from build123d import *

# Parameters (mm, degrees)
ESQUISSE2_W             = 5
ESQUISSE2_H             = 12.5
ESQUISSE3_R             = 2
ENL_V_MAT_EXTRU_1_DEPTH = 36
ESQUISSE4_R             = 3
ENL_V_MAT_EXTRU_2_DEPTH = 36
ESQUISSE5_W             = 30
ESQUISSE5_H             = 3.421913798


with BuildPart() as part:
    # Esquisse1 → Révolution1 (revolve)
    with BuildSketch(Plane.XY):
        Polygon((0, 34), (0, 0), (8, 0), (8, 40), (3, 40), (3, 39), (-27, 39), (-27, 40), (-32, 40), (-32, 34), align=None)
    revolve(axis=Axis((-49.644499027, 0, 0), (1, 0, 0)))

    # Esquisse2 → Enlèvement de matière-Révolution1 (revolve, cut)
    with BuildSketch(Plane.XY):
        with Locations((5.5, 6.25)):
            Rectangle(ESQUISSE2_W, ESQUISSE2_H)
    revolve(axis=Axis((0, 0, 0), (1, 0, 0)), mode=Mode.SUBTRACT)

    # Esquisse3 → Enlèv. mat.-Extru.1 (cut, through all)
    with BuildSketch(Plane(origin=(3, 0, 0), x_dir=(0, 0, -1), z_dir=(1, 0, 0))):
        with Locations((4.75, 8.227241336)):
            Circle(ESQUISSE3_R)
        with Locations((-4.75, 8.227241336)):
            Circle(ESQUISSE3_R)
        with Locations((4.75, -8.227241336)):
            Circle(ESQUISSE3_R)
        with Locations((-4.75, -8.227241336)):
            Circle(ESQUISSE3_R)
    extrude(amount=-ENL_V_MAT_EXTRU_1_DEPTH, mode=Mode.SUBTRACT)

    # Esquisse4 → Enlèv. mat.-Extru.2 (cut, through all)
    with BuildSketch(Plane(origin=(3, 0, 0), x_dir=(0, 0, -1), z_dir=(1, 0, 0))):
        Circle(ESQUISSE4_R)
    extrude(amount=-ENL_V_MAT_EXTRU_2_DEPTH, mode=Mode.SUBTRACT)

    # Esquisse5 → Révolution2 (revolve)
    with BuildSketch(Plane.XY):
        with Locations((-12, 40.710956899)):
            Rectangle(ESQUISSE5_W, ESQUISSE5_H)
    revolve(axis=Axis((0, 0, 0), (-1, 0, 0)))


solid = part.part
Can you work these out from the model? Positions are in its coordinate system, mm. A direction names the side the tool comes from. Coordinates: 2 decimals unless noted, no trailing zeros. Order: outer loops, then holes, each group sorted by start corner. A loop starts at its lowest first (then second) coordinate and runs counter-clockwise, first axis right, second up. Notation, with made-up numbers: M 39.5,5.5 L 95.5,5.5 A23 ccw 95.5,42.5 Z; hole C 33.5,77 d5. An arc over 180 degrees is marked long. Write item = value, one per line.
(1) Suppose I cut it at D-D on z = 31.5. Please give me the cut outline in (x, y), plus the area to 3 significant figures.
Results are:
outline = M -32,-24.65 L -27,-24.65 L -27,-28.41 L 3,-28.41 L 3,-24.65 L 8,-24.65 L 8,24.65 L 3,24.65 L 3,28.41 L -27,28.41 L -27,24.65 L -32,24.65 L -32,12.8 L 0,12.8 L 0,-12.8 L -32,-12.8 Z
area = 1,380 mm2
(2) If we mould it in two halves opening along Z, with no side actions, what happens to faces 4 (the face through (1.52, -9.44, 6.34)), 5 (the face through (5.46, -8.67, -39.05)), 6 (the face through (-32, -18, -29.4))? For each: pulls with the +Z half, pulls with the -Z half, needs draft (parallel to the pull), parting line crosses it, or undercut.
Results are:
face_4 = undercut
face_5 = parting line crosses it
face_6 = needs draft
(3) For faces 1 (the face through (3, -31.2, -25.3)), 2 (the face through (8, 9, 9)), 3 (the face through (0, 7, 0)), which set-ups out of +Z, -Z, +X, -X, +Y, -Y let a thin tool reach every point of the face, with its end or its side?
Results are:
face_1 = +X
face_2 = +Z, -Z, +X, +Y, -Y
face_3 = -X
(4) Suppose I cut it at C-C on x = -3. Please give me the cut outline in (y, z), plus the area to 3 significant figures.
Results are:
outline = C 0,0 d84.84; hole C 0,0 d68
area = 2,020 mm2
(5) I need wall thicknesses on line 1 along Y through (x, z) = (0.7, 4.75); line 2 along Y through (x, z) = (1, -4); line 3 along X through (y, z) = (17.5, 37.5). Which ranges of each line are inside material? Lowest first, please. Write a range as [from, to].
Results are:
line_1 = [-42.16, -10.23], [-6.23, 6.23], [10.23, 42.16]
line_2 = [-42.23, -10.08], [-6.37, 6.37], [10.08, 42.23]
line_3 = [-27, 3]
(6) Suppose I cut it at A-A on y = 0. Please give me the cut outline in (x, z).
Results are:
outline = M -32,-40 L -27,-40 L -27,-42.42 L 3,-42.42 L 3,-40 L 8,-40 L 8,-12.5 L 3,-12.5 L 3,-3 L 0,-3 L 0,-34 L -32,-34 Z; M -32,34 L 0,34 L 0,3 L 3,3 L 3,12.5 L 8,12.5 L 8,40 L 3,40 L 3,42.42 L -27,42.42 L -27,40 L -32,40 Z
(7) For pin 1 Ø3 at (y, z) = (15.5, -28.5) entering from -X; pin 2 Ø1 at (y, z) = (-31.5, -12.5) entering from -X; pin 3 Ø7.5 at (y, z) = (6, -2.5) entering from +X; pin 4 Ø3 at (x, z) = (-21, 33.5) entering from +Y, each with a flat end and sliding along its axis, tell me the tip position at first contact or that it passes through.
Results are:
pin_1 = 0
pin_2 = -32
pin_3 = 3
pin_4 = 27.85
